```python
from build123d import *

# Parameters (mm, degrees)
SKETCH034_R          = 2.45
PAD017_DEPTH         = 1.6
SKETCH035_R          = 2.6
PAD018_DEPTH         = 6
SKETCH061_W          = 1.7771358599
SKETCH061_H          = 3.8
POCKET023_DEPTH      = 1.6
POCKET023_DEPTH_BACK = 3


with BuildPart() as part:
    # Sketch034 → Pad017 (new body)
    with BuildSketch(Plane.YZ.offset(8.7)):
        with BuildLine():
            ThreePointArc((-6, 6), (-7.4371881489, -9.1), (-6, -24.2))
            Line((-6, -24.2), (0, -24.2))
            ThreePointArc((0, -24.2), (4.2426406871, -22.4426406871), (6, -18.2))
            Line((6, 0), (6, -18.2))
            ThreePointArc((6, 0), (4.2426406871, 4.2426406871), (0, 6))
            Line((-6, 6), (0, 6))
        make_face()
        Circle(SKETCH034_R, mode=Mode.SUBTRACT)
        with Locations((0, -18.2)):
            Circle(SKETCH034_R, mode=Mode.SUBTRACT)
    extrude(amount=-PAD017_DEPTH)

    # Sketch035 → Pad018 (join)
    with BuildSketch(Plane.YZ.offset(8.7)):
        with BuildLine():
            ThreePointArc((5.8114989668, -16.707860677), (3.6774423219, -13.4590699257), (0, -12.2))
            Line((-7.3771358599, -12.2), (0, -12.2))
            ThreePointArc((-6, 6), (-7.2090239265, -3.0606187573), (-7.3771358599, -12.2))
            Line((-6, 6), (0, 6))
            ThreePointArc((6, 0), (4.2426406871, 4.2426406871), (0, 6))
            Line((6, 0), (6, -17.4420237293))
            Line((6, -17.4420237293), (5.8114989668, -16.707860677))
        make_face()
        Circle(SKETCH035_R, mode=Mode.SUBTRACT)
    extrude(amount=PAD018_DEPTH)

    # Sketch061 → Pocket023 (cut, two sides)
    with BuildSketch(Plane.YZ.offset(8.7)) as pocket023_sk:
        with BuildLine():
            ThreePointArc((-6.3244944235, -22.4), (-6.167388681, -23.3009268767), (-6, -24.2))
            Line((-6, -24.2), (-4.8, -24.2))
            Line((-4.8, -24.2), (-4.8, -22.4))
            Line((-4.8, -22.4), (-6.3244944235, -22.4))
        make_face()
        with Locations((-5.68856793, -9.1)):
            Rectangle(SKETCH061_W, SKETCH061_H)
        with BuildLine():
            Line((-6, 6), (-4.8, 6))
            Line((-4.8, 6), (-4.8, 4.2))
            Line((-4.8, 4.2), (-6.3244944235, 4.2))
            ThreePointArc((-6, 6), (-6.167388681, 5.1009268767), (-6.3244944235, 4.2))
        make_face()
    extrude(amount=-POCKET023_DEPTH, mode=Mode.SUBTRACT)
    extrude(pocket023_sk.sketch, amount=POCKET023_DEPTH_BACK, mode=Mode.SUBTRACT)


with BuildPart() as part_1:
    # Body016 placement: moved
    add(part.part.moved(Location((0, -72.6064407756, 0))))


solid = part_1.part
```
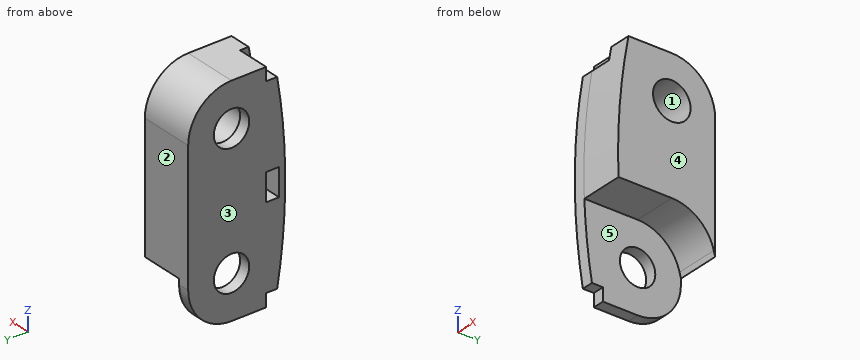
Part model, mm, in its own coordinate system. Face numbers are marked on the shaded views. A direction names the side the tool comes from. Give positions to 0.01 mm unless a question says otherwise; leave off trailing zeros. Write each loop counter-clockwise with the first axis right and the second up, starting at its lowest first coordinate (ties: lowest second). Pieces come first, ordered by that corner, then holes. Notation, with made-up numbers: (56.5, -8.5) -> (78.5, -8.5) arc R10 cw to (78.5, 1.5) -> close; hole circle Ø1 at (34, 12). An arc over 180 degrees is marked (long way). Put each result on its own line as item: value. Start each with the question number.
Item 1: Pull direction Y, two halves, no side cores. Call the marked faces 1, 2 and 3: pulls with the +Y half, pulls with the -Y half, needs draft (parallel to the pull), parting line crosses it, or undercut.
Item 2: Which spindle directions (+Z, -Z, +X, -X, +Y, -Y) get a long thin tool onto all of the face, cutting with end or side? Do the marked faces 4 and 5. Say none if no direction does.
Item 3: Wall check: L1, parallel to X at y = -74.5, z = -15; L2, parallel to Z at x = 9.75, y = -78.5; L3, parallel to Z at x = 8.25, y = -71. Give the ranges that are in metal, low to high. Write a range as [from, to].
Item 4: Cut at B-B (z = -0.5). List the corners of the cut face in (x, y).
Item 5: Cut at D-D (y = -71). List the corners of the cut face in (x, z).
Item 6: Cut at A-A (x = 11.25). List the corners of the cut face in (y, z), then the cut area to 3 significant figures.
Item 7: Pin check, flat tips, straight feed: pin 1 Ø1.8 at (x, y) = (10.5, -75) entering from -Z; pin 2 Ø0.8 at (x, y) = (7.5, -78.5) entering from -Z; pin 3 Ø2 at (x, y) = (9.5, -69.5) entering from +Z; pin 4 Ø4 at (y, z) = (-72.61, 0) entering from +X. Stop position of each tip, or through.
Item 8: Cut at C-C (x = 12.5). List the corners of the cut face in (y, z), then the cut area to 3 significant figures.
Answer list:
1. face 1: undercut
1. face 2: pulls with the +Y half
1. face 3: needs draft
2. face 4: +Z, -Z, +X, +Y, -Y
2. face 5: -Z, +X, -Y
3. L1: x = [7.1, 8.7]
3. L2: z = [-12.2, -11], [-7.2, 4.2]
3. L3: z = [-23.98, -20.05], [-16.35, -1.85], [1.85, 5.78]
4. outline: (7.1, -79.58) -> (14.7, -79.58) -> (14.7, -75.16) -> (8.7, -75.16) -> (8.7, -75) -> (7.1, -75) -> close; (7.1, -70.21) -> (8.7, -70.21) -> (8.7, -70.05) -> (14.7, -70.05) -> (14.7, -66.61) -> (7.1, -66.61) -> close
5. outline: (7.1, -23.98) -> (8.7, -23.98) -> (8.7, -20.05) -> (7.1, -20.05) -> close; (7.1, -16.35) -> (8.7, -16.35) -> (8.7, -12.42) -> (14.7, -12.42) -> (14.7, -2.04) -> (8.7, -2.04) -> (8.7, -1.85) -> (7.1, -1.85) -> close; (7.1, 1.85) -> (8.7, 1.85) -> (8.7, 2.04) -> (14.7, 2.04) -> (14.7, 5.78) -> (7.1, 5.78) -> close
6. outline: (-79.98, -12.2) -> (-72.61, -12.2) arc R6 cw to (-66.79, -16.71) -> (-66.61, -17.44) -> (-66.61, 0) arc R6 ccw to (-72.61, 6) -> (-77.41, 6) -> (-77.41, 4.2) -> (-78.93, 4.2) arc R80.04 ccw to start; hole (-79.18, -11) -> (-77.41, -11) -> (-77.41, -7.2) -> (-79.18, -7.2) -> close; hole circle Ø5.2 at (-72.61, 0)
6. area: 207 mm2
7. pin 1: stops at z = -12.2
7. pin 2: stops at z = -22.4
7. pin 3: stops at z = 5.62
7. pin 4: passes through
8. outline: (-79.98, -12.2) -> (-72.61, -12.2) arc R6 cw to (-66.79, -16.71) -> (-66.61, -17.44) -> (-66.61, 0) arc R6 ccw to (-72.61, 6) -> (-78.61, 6) arc R80.04 ccw to start; hole circle Ø5.2 at (-72.61, 0)
8. area: 216 mm2
